from build123d import *

# Parameters (mm, degrees)
SKETCH_1_W          = 100
SKETCH_1_H          = 70
EXTRUDE_1_DEPTH     = 20
SKETCH_2_R          = 10
EXTRUDE_2_DEPTH     = 30
SKETCH_3_W          = 20
SKETCH_3_H          = 30
EXTRUDE_3_DEPTH     = 30
CUT_EXTRUDE_1_DEPTH = 126.39936204


with BuildPart() as part:
    # 草圖1 → 填料-伸長1 (new body)
    with BuildSketch(Plane.XY):
        Rectangle(SKETCH_1_W, SKETCH_1_H)
    extrude(amount=EXTRUDE_1_DEPTH)

    # 草圖2 → 填料-伸長2 (add)
    with BuildSketch(Plane.XY.offset(20)):
        with BuildLine():
            Line((25.617376915, 20), (40, 20))
            Line((40, 20), (40, -20))
            Line((40, -20), (25.617376915, -20))
            ThreePointArc((25.617376915, -20), (0, -32.5), (-25.617376915, -20))
            Line((-25.617376915, -20), (-40, -20))
            Line((-40, -20), (-40, 20))
            Line((-40, 20), (-25.617376915, 20))
            ThreePointArc((-25.617376915, 20), (0, 32.5), (25.617376915, 20))
        make_face()
        Circle(SKETCH_2_R, mode=Mode.SUBTRACT)
    extrude(amount=EXTRUDE_2_DEPTH)

    # 草圖3 → 填料-伸長3 (add)
    with BuildSketch(Plane.XY.offset(50)):
        with Locations((30, 0)):
            Rectangle(SKETCH_3_W, SKETCH_3_H)
        with Locations((-30, 0)):
            Rectangle(SKETCH_3_W, SKETCH_3_H)
    extrude(amount=EXTRUDE_3_DEPTH)

    # 草圖4 → 除料-伸長1 (cut, through all)
    with BuildSketch(Plane.ZY.offset(40)):
        with BuildLine():
            ThreePointArc((90, 0), (87.071067812, 7.071067812), (80, 10))
            Line((80, 10), (80, -10))
            ThreePointArc((80, -10), (87.071067812, -7.071067812), (90, 0))
        make_face()
        with BuildLine():
            Line((80, -10), (80, 10))
            ThreePointArc((80, 10), (70, 0), (80, -10))
        make_face()
    extrude(amount=-CUT_EXTRUDE_1_DEPTH, mode=Mode.SUBTRACT)


solid = part.part
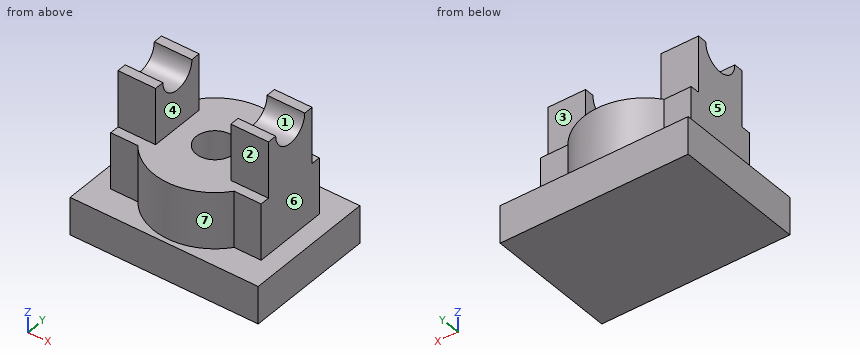
Can you work these out from the model? Positions are in its coordinate system, mm. Face numbers are marked on the shaded views. A direction names the side the tool comes from. Coordinates: 2 decimals unless noted, no trailing zeros. Write each loop counter-clockwise with the first axis right and the second up, starting at its lowest first coordinate (ties: lowest second). Pieces come first, ordered by that corner, then holes. Notation, with made-up numbers: (53, -27.5) -> (98, -27.5) arc R22 cw to (98, 6.5) -> close; hole circle Ø8 at (28, 55.25). An arc over 180 degrees is marked (long way). Write each question's results on one line, items separated by ' | '. Start each with the question number.
Q1. We'd pull the mould along Y, two halves only. Please class the marked faces 1, 2, 3 and 4: +Y half, -Y half, draft (parallel to the pull), parting line (faces both ways), or undercut.
Q2. On a 3-axis mill with a long thin cutter (end or side, diameter ignored), from which of +Z, -Z, +X, -X, +Y, -Y can I reach the whole of each face in a straight line? I mean the marked faces 5, 6 and 7. Say none if no direction works.
Q3. Imagine slicing it at C-C (z = 73). Write out the boundary of the cut face in (x, y).
Q4. If I drill on probe 1 along Y at (x, z) = (0, 28.75); probe 2 along Z at (x, y) = (-42, -5.5); probe 3 along X at (y, z) = (13, 30.5), over which ranges is the centre line in solid material (lowest first)?
Q5. Imagine slicing it at A-A (z = 37). Write out the boundary of the cut face in (x, y), then the cut area to 3 significant figures.
Q6. I'm going to push flat-ended pins straight in: pin 1 (10 mm diameter, centred on x = 7.5, z = 46.5, fed in from +Y); pin 2 (9 mm diameter, centred on y = -3.5, z = 72.5, fed in from +X); pin 3 (8 mm diameter, centred on x = 28.5, z = 64, fed in from +Y). Where does each tip first touch, or does it pass through?
Q7. Imagine slicing it at D-D (x = 0). Write out the boundary of the cut face in (y, z).
Q8. Imagine slicing it at B-B (y = 8). Write out the boundary of the cut face in (x, z), then the cut area to 3 significant figures.
Taken from the geometry:
1) face 1: undercut | face 2: -Y half | face 3: +Y half | face 4: draft
2) face 5: +Z, -X, +Y, -Y | face 6: +Z, +X, +Y, -Y | face 7: +Z, -Y
3) outline: (-40, -15) -> (-20, -15) -> (-20, -7.14) -> (-40, -7.14) -> close; (-40, 7.14) -> (-20, 7.14) -> (-20, 15) -> (-40, 15) -> close; (20, -15) -> (40, -15) -> (40, -7.14) -> (20, -7.14) -> close; (20, 7.14) -> (40, 7.14) -> (40, 15) -> (20, 15) -> close
4) probe 1: y = -32.5 to -10, 10 to 32.5 | probe 2: z = 0 to 20 | probe 3: x = -40 to 40
5) outline: (-40, -20) -> (-25.62, -20) arc R32.5 ccw to (25.62, -20) -> (40, -20) -> (40, 20) -> (25.62, 20) arc R32.5 ccw to (-25.62, 20) -> (-40, 20) -> close; hole circle Ø20 at (0, 0) | area: 3,780 mm^2
6) pin 1: stops at y = 32.4 | pin 2: stops at x = 40 | pin 3: stops at y = 15
7) outline: (-35, 0) -> (35, 0) -> (35, 20) -> (32.5, 20) -> (32.5, 50) -> (10, 50) -> (10, 20) -> (-10, 20) -> (-10, 50) -> (-32.5, 50) -> (-32.5, 20) -> (-35, 20) -> close
8) outline: (-50, 0) -> (50, 0) -> (50, 20) -> (40, 20) -> (40, 74) -> (20, 74) -> (20, 50) -> (6, 50) -> (6, 20) -> (-6, 20) -> (-6, 50) -> (-20, 50) -> (-20, 74) -> (-40, 74) -> (-40, 20) -> (-50, 20) -> close | area: 5,000 mm^2
